```python
from build123d import *

# Parameters (mm, degrees)
ESQUISSE1_W                = 161.925
ESQUISSE1_H                = 161.925
ESQUISSE1_R                = 39.6875
BOSS_EXTRU_1_DEPTH         = 19.05
TROU_TARAUD_3_8_161_D      = 7.9375
ESQUISSE4_R                = 61.9125
ESQUISSE4_R_2              = 55.5625
ENL_V_MAT_EXTRU_1_DEPTH    = 4.7625
ESQUISSE5_R                = 50.8
ESQUISSE5_R_2              = 39.6875
BOSS_EXTRU_2_DEPTH         = 26.67
CONG_1_R                   = 9.525
TROU_TARAUD_1_2_131_REACH  = 158.932
TROU_TARAUD_1_2_131_BORE_R = 5.35813
CHANFREIN2_SIZE            = 2.38125
ESQUISSE11_R               = 53.975
ESQUISSE11_R_2             = 39.6875
BOSS_EXTRU_3_DEPTH         = 19.05
CHANFREIN4_SIZE            = 2.38125


with BuildPart() as part:
    # Esquisse1 → Boss.-Extru.1 (new body)
    with BuildSketch(Plane(origin=(0, 0, 0), x_dir=(1, 0, 0), z_dir=(0, 1, 0))):
        Rectangle(ESQUISSE1_W, ESQUISSE1_H)
        with Locations(Location((0, 0, 0), (0, 0, 270))):
            Circle(ESQUISSE1_R, mode=Mode.SUBTRACT)
        with BuildLine():
            ThreePointArc((-46.438182228, 66.320597386), (-57.249132772, 57.249132772), (-66.320597386, 46.438182228))
            ThreePointArc((-66.320597386, 46.438182228), (-64.371340998, 35.383399913), (-53.316558683, 37.332656301))
            ThreePointArc((-53.316558683, 37.332656301), (-46.02381262, 46.02381262), (-37.332656301, 53.316558683))
            ThreePointArc((-37.332656301, 53.316558683), (-35.383399913, 64.371340998), (-46.438182228, 66.320597386))
        make_face(mode=Mode.SUBTRACT)
        with BuildLine():
            ThreePointArc((66.320597386, 46.438182228), (57.249132772, 57.249132772), (46.438182228, 66.320597386))
            ThreePointArc((46.438182228, 66.320597386), (35.383399913, 64.371340998), (37.332656301, 53.316558683))
            ThreePointArc((37.332656301, 53.316558683), (46.02381262, 46.02381262), (53.316558683, 37.332656301))
            ThreePointArc((53.316558683, 37.332656301), (64.371340998, 35.383399913), (66.320597386, 46.438182228))
        make_face(mode=Mode.SUBTRACT)
        with BuildLine():
            ThreePointArc((46.438182228, -66.320597386), (57.249132772, -57.249132772), (66.320597386, -46.438182228))
            ThreePointArc((66.320597386, -46.438182228), (64.371340998, -35.383399913), (53.316558683, -37.332656301))
            ThreePointArc((53.316558683, -37.332656301), (46.02381262, -46.02381262), (37.332656301, -53.316558683))
            ThreePointArc((37.332656301, -53.316558683), (35.383399913, -64.371340998), (46.438182228, -66.320597386))
        make_face(mode=Mode.SUBTRACT)
        with BuildLine():
            ThreePointArc((-66.320597386, -46.438182228), (-57.249132772, -57.249132772), (-46.438182228, -66.320597386))
            ThreePointArc((-46.438182228, -66.320597386), (-35.383399913, -64.371340998), (-37.332656301, -53.316558683))
            ThreePointArc((-37.332656301, -53.316558683), (-46.02381262, -46.02381262), (-53.316558683, -37.332656301))
            ThreePointArc((-53.316558683, -37.332656301), (-64.371340998, -35.383399913), (-66.320597386, -46.438182228))
        make_face(mode=Mode.SUBTRACT)
    extrude(amount=-BOSS_EXTRU_1_DEPTH)

    # Trou taraudé 3/8-161 (through all)
    with Locations(Plane(origin=(0, 0, 0), x_dir=(1, 0, 0), z_dir=(0, 1, 0))):
        with Locations((-63.5, 63.5), (63.5, 63.5), (-63.5, -63.5), (63.5, -63.5)):
            Hole(TROU_TARAUD_3_8_161_D / 2)

    # Esquisse4 → Enlèv. mat.-Extru.1 (cut)
    with BuildSketch(Plane(origin=(0, 0, 0), x_dir=(1, 0, 0), z_dir=(0, 1, 0))):
        with Locations(Location((0, 0, 0), (0, 0, 270))):
            Circle(ESQUISSE4_R)
        with Locations(Location((0, 0, 0), (0, 0, 270))):
            Circle(ESQUISSE4_R_2, mode=Mode.SUBTRACT)
    extrude(amount=-ENL_V_MAT_EXTRU_1_DEPTH, mode=Mode.SUBTRACT)

    # Esquisse5 → Boss.-Extru.2 (add)
    with BuildSketch(Plane(origin=(0, 0, 0), x_dir=(1, 0, 0), z_dir=(0, 1, 0))):
        with Locations(Location((0, 0, 0), (0, 0, 270))):
            Circle(ESQUISSE5_R)
        with Locations(Location((0, 0, 0), (0, 0, 270))):
            Circle(ESQUISSE5_R_2, mode=Mode.SUBTRACT)
    extrude(amount=BOSS_EXTRU_2_DEPTH)

    # Congé1
    cong_1_edges = [part.edges().sort_by_distance(p)[0] for p in [
        (80.9625, -9.525, 80.9625),
        (-80.9625, -9.525, 80.9625),
        (-80.9625, -9.525, -80.9625),
        (80.9625, -9.525, -80.9625),
    ]]
    fillet(cong_1_edges, radius=CONG_1_R)

    # Trou taraudé 1/2-131 bore → Trou taraudé 1/2-131 (cut, up to next)
    with BuildSketch(Plane.XY.offset(50.8), mode=Mode.PRIVATE) as trou_taraud_1_2_131_sk1:
        with Locations((0, 13.97)):
            Circle(TROU_TARAUD_1_2_131_BORE_R)
    trou_taraud_1_2_131_tool1 = extrude(trou_taraud_1_2_131_sk1.sketch, amount=-TROU_TARAUD_1_2_131_REACH, mode=Mode.PRIVATE) & part.part
    add(trou_taraud_1_2_131_tool1.solids().sort_by_distance((0, 13.97, 50.8))[0], mode=Mode.SUBTRACT)

    # Chanfrein2
    chanfrein2_edges = [part.edges().sort_by_distance(p)[0] for p in [
        (0, 26.67, -50.8),
        (0, 26.67, -39.6875),
    ]]
    chamfer(chanfrein2_edges, length=CHANFREIN2_SIZE)

    # Esquisse11 → Boss.-Extru.3 (add)
    with BuildSketch(Plane(origin=(0, -19.05, 0), x_dir=(-1, 0, 0), z_dir=(0, -1, 0))):
        with Locations(Location((0, 0, 0), (0, 0, 90))):
            Circle(ESQUISSE11_R)
        with Locations(Location((0, 0, 0), (0, 0, 270))):
            Circle(ESQUISSE11_R_2, mode=Mode.SUBTRACT)
    extrude(amount=BOSS_EXTRU_3_DEPTH)

    # Chanfrein4
    chanfrein4_edges = [part.edges().sort_by_distance(p)[0] for p in [
        (0, -38.1, -39.6875),
    ]]
    chamfer(chanfrein4_edges, length=CHANFREIN4_SIZE)


solid = part.part
```
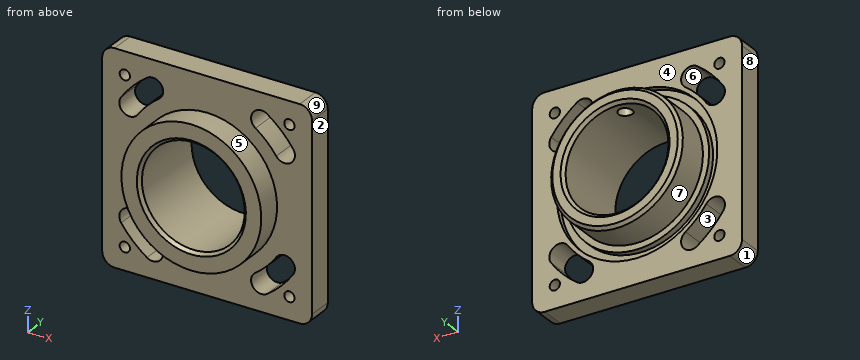
Could you check a few things on this model? Use its own coordinates, in mm. Face numbers are marked on the shaded views. A direction names the side the tool comes from. Round coordinates to 2 decimals unless told otherwise and drop trailing zeros. Answer as CSV lines item,"result".
1) For pin 1 Ø3 at (y, z) = (12, 52.5) entering from +X; pin 2 Ø9 at (x, z) = (-63.5, 63.5) entering from +Y; pin 3 Ø2 at (y, z) = (7.5, 8) entering from -X; pin 4 Ø9 at (x, z) = (63.5, -63.5) entering from -Y, each with a flat end and sliding along its axis, tell me the tip position at first contact or that it passes through.
From the geometry:
pin 1,"through"
pin 2,"y = 0"
pin 3,"x = -50.32"
pin 4,"y = -19.05"
2) Which directions (+Z, -Z, +X, -X, +Y, -Y) give clear straight access to the entire face, cutting with the end or side of a thin tool? Please do the marked faces 1, 2, 3, 4 and 5.
From the geometry:
face 1,"-Z, -X, +Y, -Y"
face 2,"+Z, -Z, +X, +Y, -Y"
face 3,"+Y, -Y"
face 4,"+Y"
face 5,"-Y"
3) If I drill on probe 1 along Z at (x, y) = (-63.5, -11.25); probe 2 along X at (y, z) = (-17, -44.5); probe 3 along Z at (x, y) = (66.5, -13), over which ranges is the centre line in solid material (lowest first)?
From the geometry:
probe 1,"-80.96 to -67.47, -59.53 to -50.23, -34.85 to 34.85, 50.23 to 59.53, 67.47 to 80.96"
probe 2,"-80.96 to -67.31, -47.5 to 47.5, 67.31 to 80.96"
probe 3,"-80.96 to -66.1, -60.9 to -46.17, -37.6 to 37.6, 46.17 to 60.9, 66.1 to 80.96"
4) We'd pull the mould along Z, two halves only. Please class the marked faces 6, 7, 8 and 9: released by +Z, released by -Z, zero draft, split by the parting line, or undercut.
From the geometry:
face 6,"undercut"
face 7,"split by the parting line"
face 8,"zero draft"
face 9,"released by +Z"
